```python
from build123d import *

# Parameters (mm, degrees)
SKETCH1_W               = 203.2
SKETCH1_H               = 116.84
BOSS_EXTRUDE1_DEPTH     = 5.08
FILLET1_R               = 6.35
SKETCH2_W               = 10.16
SKETCH2_H               = 5.08
CUT_EXTRUDE1_DEPTH      = 1
CUT_EXTRUDE1_DEPTH_BACK = 6.08
SKETCH3_W               = 17.4625
SKETCH3_H               = 5.08
CUT_EXTRUDE2_DEPTH      = 10.16


with BuildPart() as part:
    # Sketch1 → Boss-Extrude1 (new body)
    with BuildSketch(Plane.XY):
        Rectangle(SKETCH1_W, SKETCH1_H)
        Polygon((80.556430234, 48.26), (0, 5.744106266), (-80.556430234, 48.26), align=None, mode=Mode.SUBTRACT)
        Polygon((-91.44, 42.515893734), (-10.883569766, 0), (-91.44, -42.515893734), align=None, mode=Mode.SUBTRACT)
        Polygon((-80.556430234, -48.26), (0, -5.744106266), (80.556430234, -48.26), align=None, mode=Mode.SUBTRACT)
        Polygon((91.44, -42.515893734), (10.883569766, 0), (91.44, 42.515893734), align=None, mode=Mode.SUBTRACT)
    extrude(amount=BOSS_EXTRUDE1_DEPTH)

    # Fillet1
    fillet1_edges = [part.edges().sort_by_distance(p)[0] for p in [
        (-91.44, 42.515893734, 2.54),
        (-91.44, -42.515893734, 2.54),
        (-10.883569766, 0, 2.54),
        (-80.556430234, -48.26, 2.54),
        (80.556430234, -48.26, 2.54),
        (0, -5.744106266, 2.54),
        (80.556430234, 48.26, 2.54),
        (-80.556430234, 48.26, 2.54),
        (0, 5.744106266, 2.54),
        (91.44, -42.515893734, 2.54),
        (91.44, 42.515893734, 2.54),
        (10.883569766, 0, 2.54),
    ]]
    fillet(fillet1_edges, radius=FILLET1_R)

    # Sketch2 → Cut-Extrude1 (cut, two sides)
    with BuildSketch(Plane.XY.offset(5.08)) as cut_extrude1_sk:
        with Locations((-76.2, 48.26)):
            Rectangle(SKETCH2_W, SKETCH2_H)
        with Locations((76.2, 48.26)):
            Rectangle(SKETCH2_W, SKETCH2_H)
    extrude(amount=CUT_EXTRUDE1_DEPTH, mode=Mode.SUBTRACT)
    extrude(cut_extrude1_sk.sketch, amount=-CUT_EXTRUDE1_DEPTH_BACK, mode=Mode.SUBTRACT)

    # Sketch3 → Cut-Extrude2 (cut)
    with BuildSketch(Plane.XY.offset(5.08)):
        with Locations((-92.86875, -55.88)):
            Rectangle(SKETCH3_W, SKETCH3_H)
        with Locations((-57.94375, -55.88)):
            Rectangle(SKETCH3_W, SKETCH3_H)
    extrude(amount=-CUT_EXTRUDE2_DEPTH, mode=Mode.SUBTRACT)


solid = part.part
```
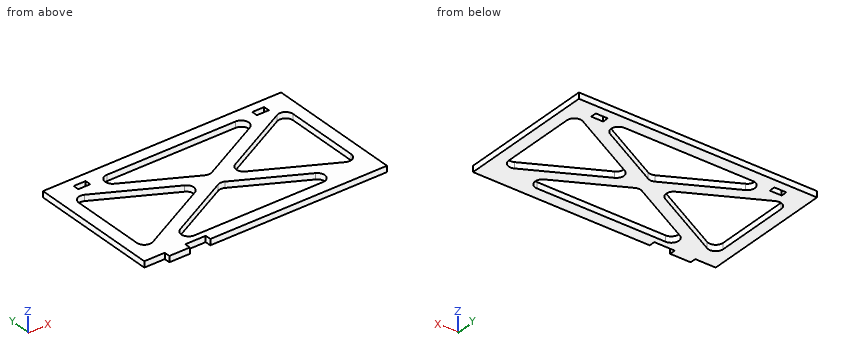
Can you work these out from the model? Positions are in its coordinate system, mm. Give positions to 0.01 mm unless a question says otherwise; leave off trailing zeros. Order: outer loops, then holes, each group sorted by start corner. A loop starts at its lowest first (then second) coordinate and runs counter-clockwise, first axis right, second up. Notation, with made-up numbers: M 56.25,20.5 L 92.25,20.5 A34 ccw 92.25,51.5 Z; hole C 41.5,84.25 d2. An arc over 180 degrees is marked long. Write item = value, one per line. Start each with the question number.
Q1. Suppose I cut it at A-A (x = 88.5). Write out the boundary of the cut face in (y, z).
Q2. Suppose I cut it at D-D (y = -42). Write out the boundary of the cut face in (x, z).
Q3. I need wall thicknesses on probe 1 along X at (y, z) = (26.5, 1.65); probe 2 along X at (y, z) = (-16.5, 1.85); probe 3 along Y at (x, z) = (85.5, 2.6). Which ranges of each line are inside material? Lowest first, please. Write a range as [from, to].
Q4. Will these pins go through, and if not, where does the flat tip stop? pin 1 Ø10 at (x, y) = (-49, -42.5) entering from +Z; pin 2 Ø12 at (x, y) = (-5, 43) entering from -Z; pin 3 Ø1.5 at (y, z) = (-56, 2) entering from -X.
Q5. Suppose I cut it at C-C (x = 31.5). Write out the boundary of the cut face in (y, z).
Q6. Suppose I cut it at B-B (y = -22). Write out the boundary of the cut face in (x, z), plus the area to 3 significant figures.
Check result:
q1.outline = M -58.42,0 L -37.34,0 L -37.34,5.08 L -58.42,5.08 Z; M 37.34,0 L 58.42,0 L 58.42,5.08 L 37.34,5.08 Z
q2.outline = M -101.6,0 L -61.27,0 L -61.27,5.08 L -101.6,5.08 Z; M 61.27,0 L 101.6,0 L 101.6,5.08 L 61.27,5.08 Z
q3.probe_1 = [-101.6, -91.44], [-61.09, -39.33], [39.33, 61.09], [91.44, 101.6]
q3.probe_2 = [-101.6, -91.44], [-42.15, -20.38], [20.38, 42.15], [91.44, 101.6]
q3.probe_3 = [-58.42, -38.32], [38.32, 58.42]
q4.pin_1 = through
q4.pin_2 = 0
q4.pin_3 = -84.14
q5.outline = M -58.42,0 L -48.26,0 L -48.26,5.08 L -58.42,5.08 Z; M -22.37,0 L -10.88,0 L -10.88,5.08 L -22.37,5.08 Z; M 10.88,0 L 22.37,0 L 22.37,5.08 L 10.88,5.08 Z; M 48.26,0 L 58.42,0 L 58.42,5.08 L 48.26,5.08 Z
q6.outline = M -101.6,0 L -91.44,0 L -91.44,5.08 L -101.6,5.08 Z; M -52.57,0 L -30.8,0 L -30.8,5.08 L -52.57,5.08 Z; M 30.8,0 L 52.57,0 L 52.57,5.08 L 30.8,5.08 Z; M 91.44,0 L 101.6,0 L 101.6,5.08 L 91.44,5.08 Z
q6.area = 324 mm2
